```python
from build123d import *

# Parameters (mm, degrees)
CROQUIS1_R                                           = 40.1
SALIENTE_EXTRUIR1_DEPTH                              = 3.95
CROQUIS2_R                                           = 42.75
SALIENTE_EXTRUIR2_DEPTH                              = 3.6
REFRENTADO_PARA_TORNILLO_CON_CABEZA_TRON_D           = 4.5
REFRENTADO_PARA_TORNILLO_CON_CABEZA_TRON_CBORE_D     = 9
REFRENTADO_PARA_TORNILLO_CON_CABEZA_TRON_CBORE_DEPTH = 3.1
SALIENTE_EXTRUIR3_DEPTH                              = 3.6
TALADRO_DE_MARGEN_PARA_M32_D                         = 3.4


with BuildPart() as part:
    # Croquis1 → Saliente-Extruir1 (new, symmetric)
    with BuildSketch(Plane.XY):
        Circle(CROQUIS1_R)
    extrude(amount=SALIENTE_EXTRUIR1_DEPTH, both=True)

    # Croquis2 → Saliente-Extruir2 (add)
    with BuildSketch(Plane.XY.offset(3.95)):
        Circle(CROQUIS2_R)
    extrude(amount=SALIENTE_EXTRUIR2_DEPTH)

    # Refrentado para tornillo con cabeza troncocónica de M41 (through all)
    with Locations(Plane.XY.offset(7.55)):
        with Locations((0, 27), (23.382685902, -13.5), (-23.382685902, -13.5)):
            CounterBoreHole(REFRENTADO_PARA_TORNILLO_CON_CABEZA_TRON_D / 2, REFRENTADO_PARA_TORNILLO_CON_CABEZA_TRON_CBORE_D / 2, REFRENTADO_PARA_TORNILLO_CON_CABEZA_TRON_CBORE_DEPTH)

    # Croquis6 → Saliente-Extruir3 (add)
    with BuildSketch(Plane(origin=(0, 0, -3.95), x_dir=(-1, 0, 0), z_dir=(0, 0, -1))):
        Polygon((5, 20), (5, 2.886751346), (19.820508076, -5.669872981), (14.820508076, -14.330127019), (0, -5.773502692), (-14.820508076, -14.330127019), (-19.820508076, -5.669872981), (-5, 2.886751346), (-5, 20), align=None)
    extrude(amount=SALIENTE_EXTRUIR3_DEPTH)

    # Taladro de margen para M32 (through all)
    with Locations(Plane.XY.offset(7.55)):
        with Locations((13.393920133, 32.335783638), (32.335783638, 13.393920133), (32.335783638, -13.393920133), (13.393920133, -32.335783638), (-13.393920133, -32.335783638), (-32.335783638, -13.393920133), (-32.335783638, 13.393920133), (-13.393920133, 32.335783638)):
            Hole(TALADRO_DE_MARGEN_PARA_M32_D / 2)


solid = part.part
```
The model under review builds one solid part; all positions refer to its coordinate system, in mm. A direction names the side the tool comes from. Coordinates: 2 decimals unless noted, no trailing zeros. Write each loop counter-clockwise with the first axis right and the second up, starting at its lowest first coordinate (ties: lowest second). Pieces come first, ordered by that corner, then holes. Notation, with made-up numbers: (7.5, 21.25) -> (34.5, 21.25) arc R23 ccw to (34.5, 40.25) -> close; hole circle Ø9 at (-21, 17.5). An arc over 180 degrees is marked (long way). One line per item, written item: value. Start each with the question number.
Q1. Add section D-D, the plane x = 9. Give the boundary of the cut face in (y, z), then the cut area to 3 significant figures.
Q2. To check wall thickness, follow probe 1 along Y at (x, z) = (0, -1.5); probe 2 along Z at (x, y) = (-20.5, -10.5); probe 3 along Z at (x, y) = (-6.5, -19). State the ranges of each line that lie inside material, in increasing order.
Q3. Add section C-C, the plane z = -6. Give the boundary of the cut face in (x, y).
Q4. For faces 4 (the face through (-7.51, -10.11, -5.72)), 5 (the face through (0, 20, -6)), 6 (the face through (5, 11, -6)), 7 (the face through (2.419, 30.794, 6.022)), list the 3-axis set-ups (+Z, -Z, +X, -X, +Y, -Y) from which the entire face can be reached by the end or side of a thin tool; tool diameter is ignored.
Q5. Add section B-B, the plane z = 1. Count the separate pieces of the cut face and the enclosed holes in it, then the cut area to 3 significant figures.
Q6. The part is to be moulded in two halves that separate along X. For faces 1 (the face through (2, 25, 4.45)), 2 (the face through (-5, 12, -6)), 3 (the face through (12.51, -1.45, -5.72)), say which applies: +X half, -X half, draft (parallel to the pull), parting line (faces both ways), or undercut.
Q7. Add section A-A, the plane y = 27. Give the boundary of the cut face in (x, z), then the cut area to 3 significant figures.
Q8. Clearance check with flat-ended pins moving along their axes: P1, Ø1, axis at y = 0.5, z = 2, coming from the +X side; P2, Ø4.5, axis at x = 32.34, y = -13.39, coming from the -Z side; P3, Ø8, axis at x = 6.5, z = -6, coming from the +Y side; P4, Ø5, axis at x = 20, y = -4.5, coming from the -Z side. State where each tip first meets the part, or that it passes through.
Response:
1. outline: (-41.79, 3.95) -> (-39.08, 3.95) -> (-39.08, -3.95) -> (-10.97, -3.95) -> (-10.97, -7.55) -> (0.58, -7.55) -> (0.58, -3.95) -> (39.08, -3.95) -> (39.08, 3.95) -> (41.79, 3.95) -> (41.79, 7.55) -> (-41.79, 7.55) -> close
1. area: 960 mm²
2. probe 1: -40.1 to 24.75, 29.25 to 40.1
2. probe 2: -3.95 to 4.45
2. probe 3: -3.95 to 7.55
3. outline: (-19.82, -5.67) -> (-14.82, -14.33) -> (0, -5.77) -> (14.82, -14.33) -> (19.82, -5.67) -> (5, 2.89) -> (5, 20) -> (-5, 20) -> (-5, 2.89) -> close
4. face 4: -Z, -Y
4. face 5: -Z, +X, -X, +Y
4. face 6: -Z, +X, +Y
4. face 7: +Z
5. separate pieces: 1
5. enclosed holes: 11
5. area: 4,930 mm²
6. face 1: undercut
6. face 2: -X half
6. face 3: +X half
7. outline: (-33.14, 3.95) -> (-29.65, 3.95) -> (-29.65, -3.95) -> (-2.25, -3.95) -> (-2.25, 4.45) -> (-4.5, 4.45) -> (-4.5, 7.55) -> (-33.14, 7.55) -> close; (2.25, -3.95) -> (29.65, -3.95) -> (29.65, 3.95) -> (33.14, 3.95) -> (33.14, 7.55) -> (4.5, 7.55) -> (4.5, 4.45) -> (2.25, 4.45) -> close
7. area: 641 mm²
8. P1: x = 40.1
8. P2: z = -3.95
8. P3: y = 39.98
8. P4: z = -7.55
